```python
from build123d import *

# Parameters (mm, degrees)
CYLINDER046_R               = 1.5
CYLINDER046_DEPTH           = 10
CYLINDER046_ROLL_ANGLE      = -90
CYLINDER046_PLACEMENT_ANGLE = 41
BOX014_W                    = 5
BOX014_H                    = 11
BOX014_DEPTH                = 9
BOX014_PLACEMENT_ANGLE      = 49
BOX013_W                    = 11
BOX013_H                    = 10
BOX013_DEPTH                = 12
BOX013_PLACEMENT_ANGLE      = 49


with BuildPart() as cylinder046:
    # Cylinder046 → Cylinder046 (new body)
    with BuildSketch(Plane.XY):
        Circle(CYLINDER046_R)
    extrude(amount=CYLINDER046_DEPTH)


with BuildPart() as cylinder046_1:
    # Cylinder046 roll: moved
    add(cylinder046.part.rotate(Axis((0, 0, 0), (1, 0, 0)), CYLINDER046_ROLL_ANGLE))


with BuildPart() as cylinder046_2:
    # Cylinder046 placement: moved
    add(cylinder046_1.part.moved(Location((12, 36, -6))).rotate(Axis((12, 36, -6), (0, 0, 1)), CYLINDER046_PLACEMENT_ANGLE))


with BuildPart() as box014:
    # Box014 → Box014 (new body)
    with BuildSketch(Plane.XY):
        with Locations((2.5, 5.5)):
            Rectangle(BOX014_W, BOX014_H)
    extrude(amount=BOX014_DEPTH)


with BuildPart() as box014_1:
    # Box014 placement: moved
    add(box014.part.moved(Location((8, 32, -10))).rotate(Axis((8, 32, -10), (0, 0, -1)), BOX014_PLACEMENT_ANGLE))


with BuildPart() as cut042:
    # Box013 → Box013 (new body)
    with BuildSketch(Plane.XY):
        with Locations((5.5, 5)):
            Rectangle(BOX013_W, BOX013_H)
    extrude(amount=BOX013_DEPTH)


with BuildPart() as cut042_1:
    # Box013 placement: moved
    add(cut042.part.moved(Location((6, 35, -13))).rotate(Axis((6, 35, -13), (0, 0, -1)), BOX013_PLACEMENT_ANGLE))

    # Cut041: cut Box014
    add(box014_1.part, mode=Mode.SUBTRACT)

    # Cut042: cut Cylinder046
    add(cylinder046_2.part, mode=Mode.SUBTRACT)


solid = cut042_1.part
```
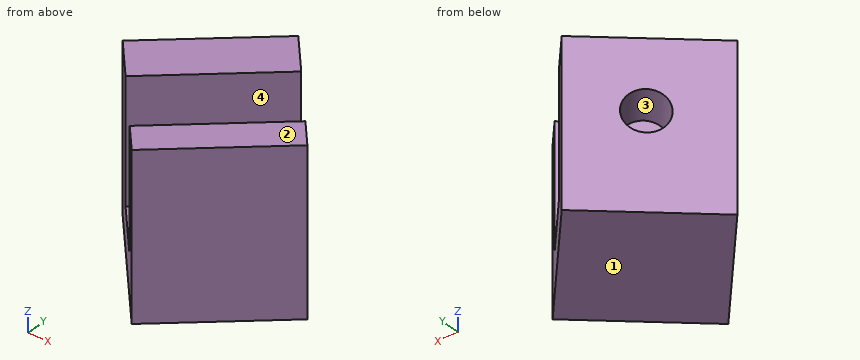
Could you check a few things on this model? Use its own coordinates, in mm. Face numbers are marked on the shaded views. Round coordinates to 2 decimals unless told otherwise and drop trailing zeros. Loops run counter-clockwise (first coordinate to the right, second up) from the corner with the lowest first, then second, coordinate; pieces in that order, holes last. Notation, with made-up numbers: (74.25, -23) - (131.25, -23) arc R27 cw to (131.25, 13) - close; hole circle Ø8 at (23.5, -11.75). An arc over 180 degrees is marked (long way). Answer in a Markdown table with one row per item. Add a question column.
(1) If we section it at D-D (z = -5): Please give me the cut outline in (x, y).
(2) If we section it at B-B (y = 32.5): Please give me the cut outline in (x, z), plus the area to 3 significant figures.
(3) I need wall thicknesses on line 1 along Y through (x, z) = (11.25, -6); line 2 along Z through (x, y) = (13.5, 34.25); line 3 along Y through (x, z) = (14.25, -3.25). Which ranges of each line are inside material? Lowest first, please.
(4) If we section it at A-A (z = -3.25): Please give me the cut outline in (x, y).
(5) If we mould it in two halves opening along Z, with no side actions, what happens to the marked faces 1, 2, 3 and 4? For each: pulls with the +Z half, pulls with the -Z half, needs draft (parallel to the pull), parting line crosses it, or undercut.
(6) If we section it at C-C (x = 18.25): Please give me the cut outline in (y, z).
(7) I'm going to push flat-ended pins straight in: pin 1 (4 mm diameter, centred on x = 8.5, y = 29.5, fed in from +Z); pin 2 (2 mm diameter, centred on y = 31.5, z = -10.5, fed in from -X); pin 3 (4 mm diameter, centred on y = 39.5, z = -6, fed in from +X). Where does each tip first touch, or does it pass through?
Model answer:
| question | item | result |
|---|---|---|
| 1 | outline | (6, 35) - (8.35, 32.3) - (15.89, 38.86) - (13.55, 41.56) - (10.76, 39.13) - (12.84, 36.73) - (11.16, 35.27) - (9.07, 37.67) - close; (11.63, 28.53) - (13.22, 26.7) - (20.76, 33.26) - (19.17, 35.09) - close |
| 2 | outline | (8.17, -13) - (19.89, -13) - (19.89, -1) - (16.2, -1) - (16.2, -10) - (8.58, -10) - (8.58, -1) - (8.17, -1) - close |
| 2 | area | 72.0 mm² |
| 3 | line 1 | y = 34.83 to 35.35, 39.15 to 39.56 |
| 3 | line 2 | z = -13 to -10 |
| 3 | line 3 | y = 27.6 to 30.81, 37.43 to 40.75 |
| 4 | outline | (6, 35) - (8.35, 32.3) - (15.89, 38.86) - (13.55, 41.56) - close; (11.63, 28.53) - (13.22, 26.7) - (20.76, 33.26) - (19.17, 35.09) - close |
| 5 | face 1 | pulls with the -Z half |
| 5 | face 2 | pulls with the +Z half |
| 5 | face 3 | undercut |
| 5 | face 4 | needs draft |
| 6 | outline | (31.07, -13) - (36.15, -13) - (36.15, -10) - (34.29, -10) - (34.29, -1) - (31.07, -1) - close |
| 7 | pin 1 | stops at z = -10 |
| 7 | pin 2 | stops at x = 8.17 |
| 7 | pin 3 | stops at x = 15.89 |
